Design review of the part built by this model. Coordinates are the model's own, in mm. A direction names the side the tool comes from. Coordinates: 2 decimals unless noted, no trailing zeros. Loops run counter-clockwise (first coordinate to the right, second up) from the corner with the lowest first, then second, coordinate; pieces in that order, holes last. Notation, with made-up numbers: M 61,-26 L 107,-26 A8 cw 107,-21 Z; hole C 87,61.25 d11. An arc over 180 degrees is marked long. Answer as a JSON object with one key per item and string values. Group by question number.
1. Insertion check: pin 1 (1.5 mm diameter, centred on x = 93, y = -3, fed in from +Z); pin 2 (5 mm diameter, centred on x = 29, y = -13, fed in from +Z); pin 3 (5 mm diameter, centred on x = 64, z = 14.625, fed in from -Y). Each pin has a flat end and moves straight along its axis. Give the tip position at first contact, or say it passes through.
2. To check wall thickness, follow probe 1 along X at (y, z) = (-12.25, -10); probe 2 along X at (y, z) = (-9, 14); probe 3 along Z at (x, y) = (64, -9.25) (3 decimals). State the ranges of each line that lie inside material, in increasing order.
3. Draft analysis for pull direction Z (two halves, no side actions). For faces 6 (the cylindrical face through (108.577, -15.046, -0.331)), 7 (the flat face through (120, -15.2, 0.1)), 8 (the cylindrical face through (59.16, -5.306, 18.394)), 9 (the cylindrical face through (60.84, -5.306, -18.394)), state which applies: +Z half, -Z half, draft (parallel to the pull), parting line (faces both ways), or undercut.
4. Machinability: for faces 1 (the cylindrical face through (101.768, -16.346, -0.36)), 2 (the flat face through (59, -19, 0)), 3 (the cylindrical face through (99.76, -14.546, -0.32)), 4 (the flat face through (35, -5, 10.25)), 5 (the cylindrical face through (64.88, -4.92, -12.94)), which of the approach directions +Z, -Z, +X, -X, +Y, -Y give a long, thin tool a straight path to every point of the face, cutting with its end or side? Answer none if there is none.
5. Consider section D-D (z = -11.5). State the section outline as (x, y) points.
6. Consider section A-A (z = 0). State the section outline as (x, y) points, then the cut area to 3 significant figures.
7. Consider section C-C (x = 6.5). State the section outline as (y, z) points (3 decimals), then the cut area to 3 significant figures.
8. Consider section B-B (x = 28). State the section outline as (y, z) points.
from build123d import *

# Parameters (mm, degrees)
R_VOLUTION1_ANGLE       = 180
ENL_V_START             = -19
ESQUISSE2_W             = 120
ESQUISSE2_H             = 50.1
ENL_V_MAT_EXTRU_1_DEPTH = 10
ESQUISSE3_W             = 146.438377439
ESQUISSE3_H             = 50.311635948
ENL_V_MAT_EXTRU_2_DEPTH = 10
ESQUISSE4_W             = 156.060048108
ESQUISSE4_H             = 43.154210134
ENL_V_MAT_EXTRU_3_DEPTH = 7
CONG_1_R                = 10
ENL_V_MAT_EXTRU_4_DEPTH = 121
ESQUISSE6_R             = 1.9
ENL_V_MAT_EXTRU_5_DEPTH = 20


with BuildPart() as part:
    # Esquisse1 → Révolution1 (revolve, symmetric)
    with BuildSketch(Plane.XY) as r_volution1_sk:
        Polygon((70.5, -15.05), (99, -15.05), (99, -14.55), (100.5, -14.55), (100.5, -15.05), (100.5, -16.35), (103, -16.35), (103, -15.05), (114, -15.05), (114, -14.55), (115.5, -14.55), (115.5, -15.05), (115.5, -16.35), (118, -16.35), (118, -15.05), (120, -15.05), (120, -25.05), (0, -25.05), (0, -15.05), (0, -9.55), (70.5, -9.55), align=None)
    revolve(axis=Axis((0, 0, 0), (1, 0, 0)), revolution_arc=R_VOLUTION1_ANGLE / 2)
    revolve(r_volution1_sk.sketch, axis=Axis((0, 0, 0), (-1, 0, 0)), revolution_arc=R_VOLUTION1_ANGLE / 2)

    # Esquisse2 → Enlèv. mat.-Extru.1 (cut)
    with BuildSketch(Plane(origin=(0, 0, 0), x_dir=(1, 0, 0), z_dir=(0, 1, 0)).offset(ENL_V_START)):
        with Locations((60, 0)):
            Rectangle(ESQUISSE2_W, ESQUISSE2_H)
    extrude(amount=-ENL_V_MAT_EXTRU_1_DEPTH, mode=Mode.SUBTRACT)

    # Esquisse3 → Enlèv. mat.-Extru.2 (cut)
    with BuildSketch(Plane.XY.offset(ENL_V_START)):
        with Locations((56.62202011, -13.21090671)):
            Rectangle(ESQUISSE3_W, ESQUISSE3_H)
    enl_v_mat_extru_2 = extrude(amount=-ENL_V_MAT_EXTRU_2_DEPTH, mode=Mode.SUBTRACT)

    # Esquisse4 → Enlèv. mat.-Extru.3 (cut)
    with BuildSketch(Plane(origin=(0, -16.324904288, -19), x_dir=(-1, 0, 0), z_dir=(0, -0.651692786, -0.758483034))):
        with Locations((-53.986796091, -2.160595236)):
            Rectangle(ESQUISSE4_W, ESQUISSE4_H)
    enl_v_mat_extru_3 = extrude(amount=-ENL_V_MAT_EXTRU_3_DEPTH, mode=Mode.SUBTRACT)

    # Symétrie1: Enlèv. mat.-Extru.2, Enlèv. mat.-Extru.3 across plane
    add(enl_v_mat_extru_2.mirror(Plane.XY), mode=Mode.SUBTRACT)
    add(enl_v_mat_extru_3.mirror(Plane.XY), mode=Mode.SUBTRACT)

    # Congé1
    cong_1_edges = [part.edges().sort_by_distance(p)[0] for p in [
        (60, -5.583646825, 19),
        (60, -5.583646825, -19),
    ]]
    fillet(cong_1_edges, radius=CONG_1_R)

    # Esquisse5 → Enlèv. mat.-Extru.4 (cut, through all)
    with BuildSketch(Plane.ZY):
        Polygon((10.25, 0), (-10.25, 0), (-10.25, -9.9), (-3, -9.9), (-3, -13.9), (3, -13.9), (3, -9.9), (10.25, -9.9), align=None)
    extrude(amount=-ENL_V_MAT_EXTRU_4_DEPTH, mode=Mode.SUBTRACT)

    # Esquisse6 → Enlèv. mat.-Extru.5 (cut, through all)
    with BuildSketch(Plane(origin=(0, 0, 0), x_dir=(1, 0, 0), z_dir=(0, 1, 0))):
        with Locations((6.5, 14.625)):
            Circle(ESQUISSE6_R)
        with Locations((64, 14.625)):
            Circle(ESQUISSE6_R)
    enl_v_mat_extru_5 = extrude(amount=-ENL_V_MAT_EXTRU_5_DEPTH, mode=Mode.SUBTRACT)

    # Symétrie2: Enlèv. mat.-Extru.5 across plane
    add(enl_v_mat_extru_5.mirror(Plane.XY), mode=Mode.SUBTRACT)


solid = part.part
Findings below:
{
 "1": {"pin 1": "stops at z = 18.99", "pin 2": "stops at z = 14.78", "pin 3": "stops at y = -13.59"},
 "2": {"probe 1": "x = 0 to 100.5, 103 to 115.5, 118 to 120", "probe 2": "x = 0 to 4.71, 8.29 to 62.21, 65.79 to 120", "probe 3": "z = -12.725 to -10.25, 10.25 to 12.725"},
 "3": {"face 6": "undercut", "face 7": "draft", "face 8": "+Z half", "face 9": "-Z half"},
 "4": {"face 1": "+Y", "face 2": "+Z, -Z, +X, -X, -Y", "face 3": "+X, +Y", "face 4": "+X, -X, +Y", "face 5": "+Y, -Y"},
 "5": {"outline": "M 0,-14.31 L 120,-14.31 L 120,-9.71 L 118,-9.71 L 118,-11.62 L 115.5,-11.62 L 115.5,-8.91 L 114,-8.91 L 114,-9.71 L 103,-9.71 L 103,-11.62 L 100.5,-11.62 L 100.5,-8.91 L 99,-8.91 L 99,-9.71 L 70.5,-9.71 L 70.5,0 L 0,0 Z"},
 "6": {"outline": "M 0,-19 L 120,-19 L 120,-15.05 L 118,-15.05 L 118,-16.35 L 115.5,-16.35 L 115.5,-14.55 L 114,-14.55 L 114,-15.05 L 103,-15.05 L 103,-16.35 L 100.5,-16.35 L 100.5,-14.55 L 99,-14.55 L 99,-15.05 L 70.5,-15.05 L 70.5,-13.9 L 0,-13.9 Z", "area": "550 mm^2"},
 "7": {"outline": "M -19,-7.473 L -12.887,-12.725 L 0,-12.725 L 0,-10.25 L -9.9,-10.25 L -9.9,-3 L -13.9,-3 L -13.9,3 L -9.9,3 L -9.9,10.25 L 0,10.25 L 0,12.725 L -12.887,12.725 L -19,7.473 Z; M -8.464,-16.525 L -8.395,-16.585 A10 ccw -1.878,-19 L 0,-19 L 0,-16.525 Z; M -8.464,16.525 L 0,16.525 L 0,19 L -1.878,19 A10 ccw -8.395,16.585 Z", "area": "256 mm^2"},
 "8": {"outline": "M -19,-7.47 L -8.39,-16.58 A10 ccw -1.88,-19 L 0,-19 L 0,-10.25 L -9.9,-10.25 L -9.9,-3 L -13.9,-3 L -13.9,3 L -9.9,3 L -9.9,10.25 L 0,10.25 L 0,19 L -1.88,19 A10 ccw -8.39,16.58 L -19,7.47 Z"}
}
